from build123d import *

# Parameters (mm, degrees)
BOSS_EXTRUDE1_DEPTH = 60
SKETCH2_R           = 2.45
CUT_EXTRUDE1_DEPTH  = 81.642544603
CUT_EXTRUDE2_DEPTH  = 81.642544603
SKETCH4_W           = 18
SKETCH4_H           = 18
SKETCH4_R           = 2.95
BOSS_EXTRUDE2_DEPTH = 10


with BuildPart() as part:
    # Sketch1 → Boss-Extrude1 (new body)
    with BuildSketch(Plane(origin=(0, 0, 0), x_dir=(1, 0, 0), z_dir=(0, 1, 0))):
        Polygon((0, 0), (38.1, 0), (38.1, -18), (18, -18), (18, -38.1), (0, -38.1), align=None)
    extrude(amount=BOSS_EXTRUDE1_DEPTH)

    # Sketch2 → Cut-Extrude1 (cut, through all)
    with BuildSketch(Plane(origin=(0, 60, 0), x_dir=(1, 0, 0), z_dir=(0, 1, 0))):
        with Locations(Location((6.35, -6.35, 0), (0, 0, 270))):
            Circle(SKETCH2_R)
        with Locations(Location((6.35, -19.05, 0), (0, 0, 270))):
            Circle(SKETCH2_R)
        with Locations(Location((6.35, -31.75, 0), (0, 0, 270))):
            Circle(SKETCH2_R)
        with Locations(Location((19.05, -6.35, 0), (0, 0, 270))):
            Circle(SKETCH2_R)
        with Locations(Location((31.75, -6.35, 0), (0, 0, 270))):
            Circle(SKETCH2_R)
    extrude(amount=-CUT_EXTRUDE1_DEPTH, mode=Mode.SUBTRACT)

    # Sketch3 → Cut-Extrude2 (cut, through all)
    with BuildSketch(Plane(origin=(0, 60, 0), x_dir=(1, 0, 0), z_dir=(0, 1, 0))):
        with BuildLine():
            Line((0, -6.35), (-3.023343313, -6.35))
            Line((-3.023343313, -6.35), (-3.023343313, 2.931868043))
            Line((-3.023343313, 2.931868043), (6.35, 2.931868043))
            Line((6.35, 2.931868043), (6.35, 0))
            ThreePointArc((6.35, 0), (1.859871939, -1.859871939), (0, -6.35))
        make_face()
    extrude(amount=-CUT_EXTRUDE2_DEPTH, mode=Mode.SUBTRACT)

    # Sketch4 → Boss-Extrude2 (add)
    # profile 1 of 2: a face of its own
    with BuildSketch(Plane(origin=(0, 0, 0), x_dir=(-1, 0, 0), z_dir=(0, -1, 0))):
        with Locations((-9, -47.1)):
            Rectangle(SKETCH4_W, SKETCH4_H)
        with Locations(Location((-9, -47.1, 0), (0, 0, 90))):
            Circle(SKETCH4_R, mode=Mode.SUBTRACT)
    # profile 2 of 2: a face of its own
    with BuildSketch(Plane(origin=(0, 0, 0), x_dir=(-1, 0, 0), z_dir=(0, -1, 0))):
        with Locations((-47.1, -9)):
            Rectangle(SKETCH4_W, SKETCH4_H)
        with Locations(Location((-47.1, -9, 0), (0, 0, 90))):
            Circle(SKETCH4_R, mode=Mode.SUBTRACT)
    extrude(amount=-BOSS_EXTRUDE2_DEPTH)


solid = part.part
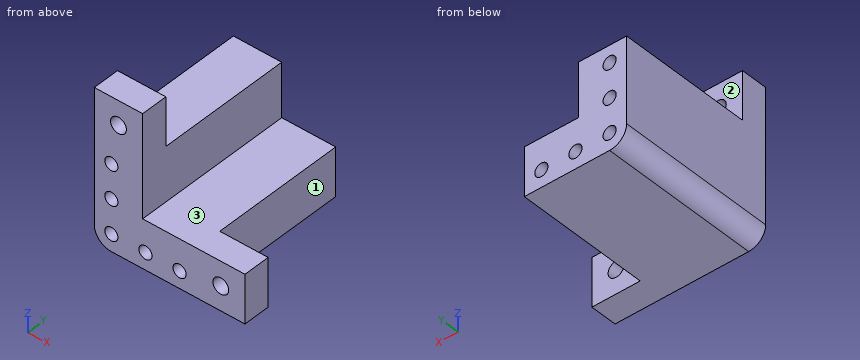
Geometry: final body of the model. Coordinates: model frame, mm. Face numbers are marked on the shaded views. A direction names the side the tool comes from. Coordinates: 2 decimals unless noted, no trailing zeros. Loops run counter-clockwise (first coordinate to the right, second up) from the corner with the lowest first, then second, coordinate; pieces in that order, holes last. Notation, with made-up numbers: (11.25, 39) - (20.25, 39) arc R18 ccw to (20.25, 71) - close; hole circle Ø2 at (-27.5, 87.5). An arc over 180 degrees is marked (long way). Put each result on its own line as item: value. Start each with the question number.
Q1. Cut plane A-A, the plane z = 19.05. Return loops of the section in (x, y).
Q2. Pin query (flat end, axial travel): pin 1 Ø5.5 at (y, z) = (33.5, 11) entering from +X; pin 2 Ø9 at (x, z) = (10.5, 43) entering from +Y; pin 3 Ø4.5 at (x, z) = (6.35, 31.75) entering from -Y; pin 4 Ø20 at (x, y) = (11.5, 27) entering from +Z. Return the tip coordinate at first contact, or that it passes through.
Q3. Cut plane B-B, the plane y = 16.5. Return loops of the section in (x, z).
Q4. Cut plane D-D, the plane z = 41. Return loops of the section in (x, y).
Q5. Line query: line 1 (X direction, y = 42, z = 6.35); line 2 (X direction, y = 39.5, z = 7.5). Output: solid intervals per line, ascending.
Q6. Set-up query: the marked faces 1, 2 and 3. Return all of +Z, -Z, +X, -X, +Y, -Y with unobstructed straight access to the full face (end or side cutting, diameter ignored); none if empty.
Q7. Cut plane C-C, the plane x = 31.75. Return loops of the section in (y, z), and give its area (3 significant figures).
Filled sheet:
1. outline: (0, 0) - (3.9, 0) - (3.9, 60) - (0, 60) - close; (8.8, 0) - (18, 0) - (18, 60) - (8.8, 60) - close
2. pin 1: x = 38.1
2. pin 2: y = 10
2. pin 3: through
2. pin 4: z = 38.1
3. outline: (0, 6.35) arc R6.35 ccw to (6.35, 0) - (38.1, 0) - (38.1, 18) - (18, 18) - (18, 38.1) - (0, 38.1) - close; hole circle Ø4.9 at (6.35, 6.35); hole circle Ø4.9 at (6.35, 19.05); hole circle Ø4.9 at (6.35, 31.75); hole circle Ø4.9 at (19.05, 6.35); hole circle Ø4.9 at (31.75, 6.35)
4. outline: (0, 0) - (18, 0) - (18, 10) - (0, 10) - close
5. line 1: 0 to 3.9, 8.8 to 16.6, 21.5 to 29.3, 34.2 to 38.1
5. line 2: 0 to 4.19, 8.51 to 16.89, 21.21 to 29.59, 33.91 to 38.1
6. face 1: +Z, -Z, +X, +Y
6. face 2: +Z, +X, -X, +Y
6. face 3: +Z, +X, +Y, -Y
7. outline: (0, 0) - (60, 0) - (60, 3.9) - (0, 3.9) - close; (0, 8.8) - (60, 8.8) - (60, 18) - (0, 18) - close
7. area: 786 mm²
